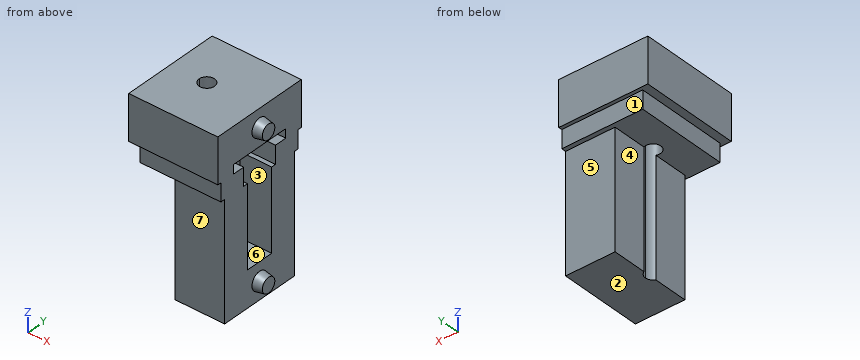
from build123d import *

# Parameters (mm, degrees)
F0_W        = 55
F0_H        = 46
F1_DEPTH    = 65
F2_W        = 35
F2_H        = 16
F3_DEPTH    = 45
F4_W        = 90
F4_H        = 51
F5_DEPTH    = 10
F6_W        = 40
F6_H        = 21
F7_DEPTH    = 10
F8_R        = 2
F9_W        = 99
F9_H        = 55
F10_DEPTH   = 25
F11_W       = 79
F11_H       = 34.5
F11_W_2     = 82.297604531
F11_H_2     = 1.4667510986
F12_DEPTH   = 5
F13_R       = 2
F14_R       = 2
F15_R       = 2
F16_R       = 2
F18_DEPTH   = 100
F19_R       = 4.25
F20_DEPTH   = 5
F21_W       = 144.5901691914
F21_H       = 163.5245941579
F10_FACE1_W = 55
F10_FACE1_H = 25
F1_FACE1_W  = 46
F1_FACE1_H  = 65
F22_DEPTH   = 49.501
F23_R       = 5
F24_DEPTH   = 5
F24_TAPER   = 10


with BuildPart() as f1:
    # F0 (on Top) → F1 (new body)
    with BuildSketch(Plane.XY):
        Rectangle(F0_W, F0_H)
    extrude(amount=F1_DEPTH)

    # F2 (on face) → F3 (cut)
    with BuildSketch(Plane.XY.offset(65)):
        Rectangle(F2_W, F2_H)
    extrude(amount=-F3_DEPTH, mode=Mode.SUBTRACT)

    # F4 (on face) → F5 (join)
    with BuildSketch(Plane.XY.offset(65)):
        Rectangle(F4_W, F4_H)
    extrude(amount=F5_DEPTH)

    # F6 (on face) → F7 (cut)
    with BuildSketch(Plane(origin=(0, 0, 65), x_dir=(1, 0, 0), z_dir=(0, 0, -1))):
        Rectangle(F6_W, F6_H)
    extrude(amount=-F7_DEPTH, mode=Mode.SUBTRACT)

    # F8
    f8_edges = [f1.edges().sort_by_distance(p)[0] for p in [
        (-20, -10.5, 70),
        (-20, 10.5, 70),
        (20, 10.5, 70),
        (20, -10.5, 70),
    ]]
    fillet(f8_edges, radius=F8_R)

    # F9 (on face) → F10 (join)
    with BuildSketch(Plane.XY.offset(75)):
        Rectangle(F9_W, F9_H)
    extrude(amount=F10_DEPTH)

    # F11 (on face) → F12 (cut)
    with BuildSketch(Plane(origin=(0, 0, 75), x_dir=(1, 0, 0), z_dir=(0, 0, -1))):
        Rectangle(F11_W, F11_H)
        with Locations((-69.0755546093, -53.2094612718)):
            Rectangle(F11_W_2, F11_H_2)
    extrude(amount=-F12_DEPTH, mode=Mode.SUBTRACT)

    # F13
    f13_edges = [f1.edges().sort_by_distance(p)[0] for p in [
        (-39.5, 17.25, 77.5),
    ]]
    fillet(f13_edges, radius=F13_R)

    # F14
    f14_edges = [f1.edges().sort_by_distance(p)[0] for p in [
        (-39.5, -17.25, 77.5),
    ]]
    fillet(f14_edges, radius=F14_R)

    # F15
    f15_edges = [f1.edges().sort_by_distance(p)[0] for p in [
        (39.5, -17.25, 77.5),
    ]]
    fillet(f15_edges, radius=F15_R)

    # F16
    f16_edges = [f1.edges().sort_by_distance(p)[0] for p in [
        (39.5, 17.25, 77.5),
    ]]
    fillet(f16_edges, radius=F16_R)

    # F17 (on face) → F18 (cut, symmetric)
    with BuildSketch(Plane(origin=(0, 0, 80), x_dir=(1, 0, 0), z_dir=(0, 0, -1))):
        with BuildLine():
            ThreePointArc((-33.5031947748, -0.0268816754), (-29.2398388853, -4.2499787461), (-25.0032797903, 0))
            ThreePointArc((-25.0032797903, 0), (-29.2667206952, 4.2499787461), (-33.5031947748, -0.0268816754))
        make_face()
    extrude(amount=F18_DEPTH, both=True, mode=Mode.SUBTRACT)

    # F19 (on face) → F20 (join)
    with BuildSketch(Plane(origin=(0, 0, 80), x_dir=(1, 0, 0), z_dir=(0, 0, -1))):
        with Locations((29.5, 0)):
            Circle(F19_R)
    extrude(amount=F20_DEPTH)

    # F21 (on Right) + F10_face1 (on face) + F1_face1 (on face) → F22 (cut, through all)
    with BuildSketch(Plane.YZ):
        with Locations((-4.733607173, 21.3217232376)):
            Rectangle(F21_W, F21_H)
    with BuildSketch(Plane(origin=(49.5, 0, 87.5), x_dir=(0, 1, 0), z_dir=(1, 0, 0))):
        Rectangle(F10_FACE1_W, F10_FACE1_H)
    with BuildSketch(Plane(origin=(27.5, 0, 32.5), x_dir=(0, 1, 0), z_dir=(1, 0, 0))):
        Rectangle(F1_FACE1_W, F1_FACE1_H)
    extrude(amount=F22_DEPTH, mode=Mode.SUBTRACT)

    # F23 (on face) → F24 (join)
    with BuildSketch(Plane.YZ):
        with Locations((0, 10)):
            Circle(F23_R)
        with Locations((0, 90)):
            Circle(F23_R)
    extrude(amount=F24_DEPTH, taper=F24_TAPER)


solid = f1.part
The model under review builds one solid part; all positions refer to its coordinate system, in mm. Face numbers are marked on the shaded views. A direction names the side the tool comes from. Coordinates: 2 decimals unless noted, no trailing zeros. Loops run counter-clockwise (first coordinate to the right, second up) from the corner with the lowest first, then second, coordinate; pieces in that order, holes last. Notation, with made-up numbers: M 68,-39 L 98,-39 A33 cw 98,-5 Z; hole C 30,77.25 d6. An arc over 180 degrees is marked long. Put each result on its own line as item: value. Start each with the question number.
Q1. Wall thickness on line 1 (Z direction, x = -33.5, y = 8); line 2 (Z direction, x = -10, y = 14); line 3 (Y direction, x = -15.5, z = 77): over which ranges is each line inside the solid? List them lowest first.
Q2. Add section C-C (z = 76.5). Write out the cut boundary in (x, y).
Q3. For the marked faces 4, 5, 6 and 7, list the 3-axis set-ups (+Z, -Z, +X, -X, +Y, -Y) from which the entire face can be reached by the end or side of a thin tool; tool diameter is ignored.
Q4. Add section D-D (z = 39). Write out the cut boundary in (x, y), and give its area (3 significant figures).
Q5. Add section B-B (x = -4). Write out the cut boundary in (y, z).
Q6. Add section A-A (x = -42). Write out the cut boundary in (y, z).
Q7. Clearance check with flat-ended pins moving along their axes: pin 1 (8 mm diameter, centred on x = -1, z = 11, fed in from +Y); pin 2 (11 mm diameter, centred on x = -11.5, z = 68, fed in from +Y); pin 3 (6 mm diameter, centred on y = -15, z = 52.5, fed in from +X). State where each tip first meets the part, or that it passes through.
Q8. The part is to be moulded in two halves that separate along Z. For the marked faces 1, 2 and 3, say which applies: +Z half, -Z half, draft (parallel to the pull), parting line (faces both ways), or undercut.
Answers:
1. line 1: z = 65 to 75, 80 to 100
1. line 2: z = 0 to 75, 80 to 100
1. line 3: y = -27.5 to -17.25, 17.25 to 27.5
2. outline: M -49.5,-27.5 L 0,-27.5 L 0,-17.25 L -37.5,-17.25 A2 cw -39.5,-15.25 L -39.5,15.25 A2 cw -37.5,17.25 L 0,17.25 L 0,27.5 L -49.5,27.5 Z
3. face 4: -Z, -X, +Y, -Y
3. face 5: -Z, +X, -X, +Y
3. face 6: +X
3. face 7: -Z, +X, -X, -Y
4. outline: M -27.5,-23 L 0,-23 L 0,-8 L -17.5,-8 L -17.5,8 L 0,8 L 0,23 L -27.5,23 L -27.5,3.87 A4.25 cw -27.5,-3.87 Z
4. area: 971 mm^2
5. outline: M -27.5,75 L -25.5,75 L -25.5,65 L -23,65 L -23,0 L 23,0 L 23,65 L 25.5,65 L 25.5,75 L 27.5,75 L 27.5,100 L -27.5,100 Z; hole M -17.25,75 L -10.5,75 L -10.5,65 L -8,65 L -8,20 L 8,20 L 8,65 L 10.5,65 L 10.5,75 L 17.25,75 L 17.25,80 L -17.25,80 Z
6. outline: M -27.5,75 L -25.5,75 L -25.5,65 L 25.5,65 L 25.5,75 L 27.5,75 L 27.5,100 L -27.5,100 Z
7. pin 1: stops at y = 23
7. pin 2: stops at y = 25.5
7. pin 3: stops at x = 0
8. face 1: draft
8. face 2: -Z half
8. face 3: undercut
